Read the model definition and answer for the solid it produces. Units are mm, in the model's axes. Round coordinates to 2 decimals unless told otherwise and drop trailing zeros. Write each loop counter-clockwise with the first axis right and the second up, starting at its lowest first coordinate (ties: lowest second). Pieces come first, ordered by that corner, then holes. Notation, with made-up numbers: (-15, 36.25) - (40, 36.25) arc R23 ccw to (40, 73.25) - close; hole circle Ø4 at (-19.75, 14.5). An arc over 180 degrees is marked (long way). Use one line per item in the form item = value. Start each with the question number.
1) The part is cut by section C-C, the plane y = -23. Give the vertices of the cut face in (x, z) (3 decimals), plus the area to 3 significant figures.
2) The part is cut by section D-D, the plane z = 296. Give the vertices of the cut face in (x, y) (3 decimals), plus the area to 3 significant figures.
3) Consider line 1 along Y through (x, z) = (0, 70) (3 decimals); line 2 along Y through (x, z) = (0.5, 119); line 3 along Y through (x, z) = (4, 345). Determine where each line is inside the solid, lowest interval first. Write a range as from..to.
4) The part is cut by section B-B, the plane z = 361. Give the vertices of the cut face in (x, y) (3 decimals), plus the area to 3 significant figures.
5) Each of these flat-tipped pins is pushed along its axis until it touches: pin 1 (5 mm diameter, centred on y = -14, z = 201.5, fed in from -X) (3 decimals); pin 2 (1.1 mm diameter, centred on x = 4.5, z = 239, fed in from +Y); pin 3 (5.5 mm diameter, centred on x = -1, y = 0, fed in from +Z). Where does it stop, or does it pass through?
6) For a pull along Z with two mould halves and no side action, classify faces 1 (the face through (3, -2, 457.2)), 2 (the face through (5.461, -23, 251)) as released by +Z, released by -Z, zero draft, split by the parting line, or undercut.
7) The part is cut by section A-A, the plane x = 0. Count the separate pieces of the cut face and the enclosed holes in it, plus the area to 3 significant figures.
from build123d import *

# Parameters (mm, degrees)
SKETCH1_R           = 3.175
BOSS_EXTRUDE1_DEPTH = 508
SKETCH2_W           = 25.4
SKETCH2_H           = 12.7
CUT_EXTRUDE1_DEPTH  = 11.922
LPATTERN1_COUNT     = 10
LPATTERN1_PITCH     = 50.8
SKETCH4_W           = 12.7
SKETCH4_H           = 30.861
SKETCH4_H_2         = 43.561
CUT_EXTRUDE2_DEPTH  = 11.922


with BuildPart() as part:
    # Sketch1 → Boss-Extrude1 (new body)
    with BuildSketch(Plane.XY):
        with BuildLine():
            Line((5.461, 0), (5.461, -38.1))
            Line((5.461, -38.1), (3.175, -38.1))
            Line((3.175, -38.1), (3.175, -4.443185344))
            ThreePointArc((3.175, -4.443185344), (-4.855985791, 2.498384078), (5.461, 0))
        make_face()
        Circle(SKETCH1_R, mode=Mode.SUBTRACT)
    extrude(amount=BOSS_EXTRUDE1_DEPTH)

    # Sketch2 → Cut-Extrude1 (cut, through all)
    with BuildSketch(Plane(origin=(5.461, 0, 0), x_dir=(0, 0, -1), z_dir=(1, 0, 0))):
        with Locations((-495.3, -0.889)):
            Rectangle(SKETCH2_W, SKETCH2_H)
    cut_extrude1 = extrude(amount=-CUT_EXTRUDE1_DEPTH, mode=Mode.SUBTRACT)

    # LPattern1: Cut-Extrude1 ×10
    with Locations(*[(0, 0, -i * LPATTERN1_PITCH) for i in range(1, LPATTERN1_COUNT)]):
        add(cut_extrude1, mode=Mode.SUBTRACT)

    # Sketch4 → Cut-Extrude2 (cut, through all)
    with BuildSketch(Plane(origin=(5.461, 0, 0), x_dir=(0, 0, -1), z_dir=(1, 0, 0))):
        with Locations((-501.65, -22.6695)):
            Rectangle(SKETCH4_W, SKETCH4_H)
        with Locations((-6.35, -16.3195)):
            Rectangle(SKETCH4_W, SKETCH4_H_2)
    extrude(amount=-CUT_EXTRUDE2_DEPTH, mode=Mode.SUBTRACT)


solid = part.part
Geometry results:
q1.outline = (3.175, 12.7) - (5.461, 12.7) - (5.461, 495.3) - (3.175, 495.3) - close
q1.area = 1,100 mm2
q2.outline = (3.175, -38.1) - (5.461, -38.1) - (5.461, -7.239) - (3.175, -7.239) - close
q2.area = 70.5 mm2
q3.line_1 = -5.461..-3.175, 3.175..5.461
q3.line_2 = -5.44..-3.14, 3.14..5.44
q3.line_3 = -38.1..-7.24
q4.outline = (3.175, -38.1) - (5.461, -38.1) - (5.461, 0) arc R5.461 ccw (long way) to (3.175, -4.443) - close; hole circle Ø6.35 at (0, 0)
q4.area = 142 mm2
q5.pin_1 = 3.175
q5.pin_2 = -7.24
q5.pin_3 = 482.6
q6.face_1 = undercut
q6.face_2 = zero draft
q7.separate_pieces = 20
q7.enclosed_holes = 0
q7.area = 1,100 mm2
